Build history of the part. All positions in model axes, mm. A direction names the side the tool comes from. Round coordinates to 2 decimals unless told otherwise and drop trailing zeros. Order: outer loops, then holes, each group sorted by start corner. A loop starts at its lowest first (then second) coordinate and runs counter-clockwise, first axis right, second up. Notation, with made-up numbers: (81, 33.25) -> (131, 33.25) arc R18 ccw to (131, 50.25) -> close; hole circle Ø3 at (-8, -4.5). An arc over 180 degrees is marked (long way). Write item = value, one per line.
from build123d import *

# Parameters (mm, degrees)
F1_DEPTH = 5
F2_R     = 4.99999


# Not quite as in the source:
# - a fillet or chamfer is up to 0.001 mm smaller than in the source, because OpenCascade refuses the exact size
# - ends of sketch curves that miss each other by under 0.0002 mm in the source are joined


with BuildPart() as f1:
    # F0 (on Top) → F1 (new body, symmetric)
    with BuildSketch(Plane.XY):
        with BuildLine():
            Line((-55, 42.9439264748), (-65, 42.9439264748))
            Line((-65, 42.9439264748), (-65, -7.0560735252))
            ThreePointArc((-65, -7.0560735252), (-60.6066017178, -17.662675243), (-50, -22.0560735252))
            Line((-50, -22.0560735252), (0, -22.0560735252))
            Line((0, -22.0560735252), (50, -22.0560729504))
            ThreePointArc((50, -22.0560729504), (60.6066017178, -17.662675243), (65, -7.0560735252))
            Line((65, -7.0560735252), (65.000000149, 42.9439264748))
            Line((65.000000149, 42.9439264748), (55, 42.9439264748))
            Line((55, 42.9439264748), (55, -7.0560735252))
            ThreePointArc((55, -7.0560735252), (53.5355343776, -10.5916079028), (50, -12.0560741922))
            Line((50, -12.0560741922), (0, -12.0560735252))
            Line((0, -12.0560735252), (-50, -12.0560735252))
            ThreePointArc((-50, -12.0560735252), (-53.5355343776, -10.5916079028), (-55.000000667, -7.0560735252))
            Line((-55.000000667, -7.0560735252), (-55, 42.9439264748))
        make_face()
    extrude(amount=F1_DEPTH, both=True)

    # F2 (radius 5 in the source; OpenCascade refuses exactly that, so slightly less here)
    f2_edges = [f1.edges().sort_by_distance(p)[0] for p in [
        (-65, 17.943926, 5),
        (-65, -7.056074, 0),
        (-60.606602, -17.662675, -5),
        (-50, -22.056074, 0),
        (-60.606602, -17.662675, 5),
        (-25, -22.056074, -5),
        (0, -22.056074, 0),
        (-25, -22.056074, 5),
        (50, -22.056073, 0),
        (60.606602, -17.662675, -5),
        (65, -7.056074, 0),
        (60.606602, -17.662675, 5),
        (55, -7.056074, 0),
        (53.535534, -10.591608, -5),
        (50, -12.056074, 0),
        (53.535534, -10.591608, 5),
        (-25, -12.056074, -5),
        (-50, -12.056074, 0),
        (-25, -12.056074, 5),
        (0, -12.056074, 0),
        (-53.535534, -10.591608, -5),
        (-55.000001, -7.056074, 0),
        (-53.535534, -10.591608, 5),
    ]]
    fillet(f2_edges, radius=F2_R)


solid = f1.part
Q1. Which spindle directions (+Z, -Z, +X, -X, +Y, -Y) get a long thin tool onto all of the face, cutting with end or side? Do faces 1 (the face through (56, 18, -3)), 2 (the face through (64, 18, -3)), 3 (the face through (-56, 18, 3)). Say none if no direction does.
Check values:
face_1 = -Z, +Y
face_2 = -Z, +X, +Y, -Y
face_3 = +Z, +Y
Q2. Probe probe 1 along X at (y, z) = (10, 0.5); probe 2 along Y at (x, z) = (15.5, 0.5); probe 3 along X at (y, z) = (6, -1.5). List the from-to ranges inside material, lowest first.
Check values:
probe_1 = -64.97 to -55.03, 55.03 to 64.97
probe_2 = -22.03 to -12.08
probe_3 = -64.77 to -55.23, 55.23 to 64.77
Q3. Flat gauge pins, fed straight in: pin 1 (2 mm diameter, centred on y = 15, z = -2, fed in from +X); pin 2 (1 mm diameter, centred on y = 7.5, z = -2.5, fed in from +X); pin 3 (1 mm diameter, centred on y = -3.5, z = 3.5, fed in from +X). Where does each tip first touch, or does it go through?
Check values:
pin_1 = 64.9
pin_2 = 64.58
pin_3 = 64
Q4. Mould opens along X. For faces 4 (the face through (56, 18, 3)), 5 (the face through (-56, 18, -3)), 6 (the face through (-64, 18, -3)), 7 (the face through (63, 18, 4)) say: released by +X, released by -X, zero draft, split by the parting line, or undercut.
Check values:
face_4 = undercut
face_5 = undercut
face_6 = released by -X
face_7 = released by +X
Q5. Cut at C-C, the plane z = -1.5. List the corners of the cut face in (x, y).
Check values:
outline = (-64.77, -7.06) arc R14.77 ccw to (-50, -21.83) -> (50, -21.83) arc R14.77 ccw to (64.77, -7.06) -> (64.77, 42.94) -> (55.23, 42.94) -> (55.23, -7.06) arc R5.23 cw to (50, -12.29) -> (-50, -12.29) arc R5.23 cw to (-55.23, -7.06) -> (-55.23, 42.94) -> (-64.77, 42.94) -> close
